The drawing under review shows one solid part. Ordinate dimensions are in mm from its lowest x, y, z. A direction names the side the tool comes from. Coordinates: 2 decimals unless noted, no trailing zeros. Order: outer loops, then holes, each group sorted by start corner. A loop starts at its lowest first (then second) coordinate and runs counter-clockwise, first axis right, second up. Notation, with made-up numbers: (34.25, -36.75) - (85.25, -36.75) arc R16 cw to (85.25, -23.75) - close; hole circle Ø9 at (82, 41.25). An arc over 180 degrees is marked (long way). Answer in a Markdown table with one row per item.
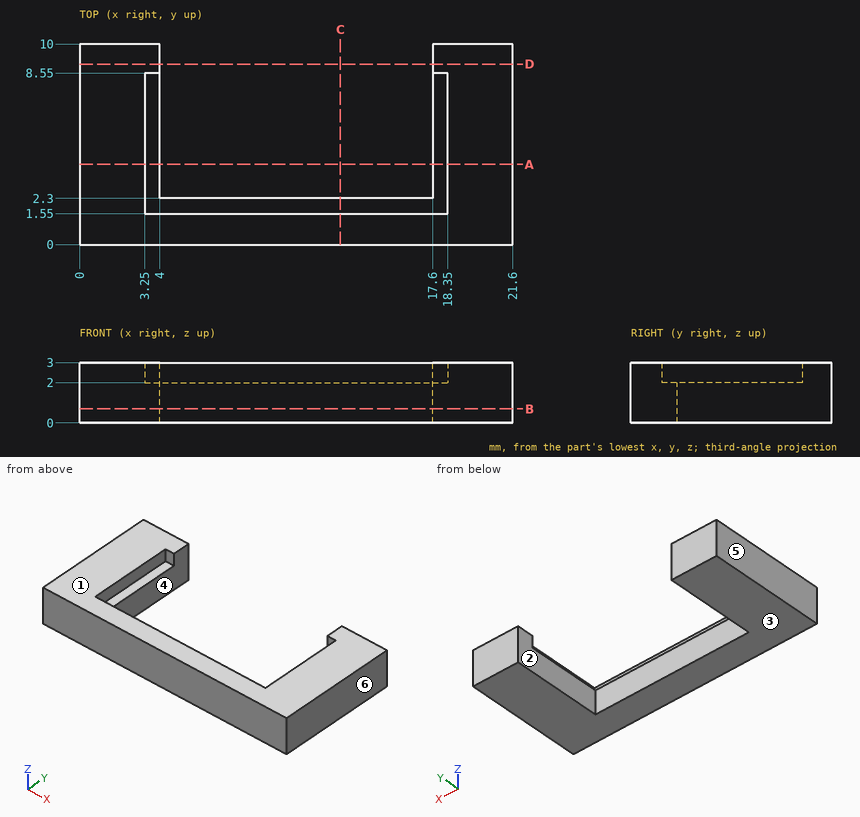
Item 1: Clearance check with a flat-ended pin moving along its axis: pin 1 Ø3.5 at (x, y) = (8.5, 4) entering from +Z. State where the tip first meets the part, or that it passes through.
Check values:
| item | result |
|---|---|
| pin 1 | z = 2 |
Item 2: We need section A-A, the plane y = 4. Write out the cut boundary in (x, z).
Check values:
| item | result |
|---|---|
| outline | (0, 0) - (4, 0) - (4, 2) - (3.25, 2) - (3.25, 3) - (0, 3) - close; (17.6, 0) - (21.6, 0) - (21.6, 3) - (18.35, 3) - (18.35, 2) - (17.6, 2) - close |
Item 3: We need section D-D, the plane y = 9. Write out the cut boundary in (x, z), then the cut area to 3 significant figures.
Check values:
| item | result |
|---|---|
| outline | (0, 0) - (4, 0) - (4, 3) - (0, 3) - close; (17.6, 0) - (21.6, 0) - (21.6, 3) - (17.6, 3) - close |
| area | 24.0 mm^2 |
Item 4: Mouldability with a two-part tool opening along X and no side actions: class the marked faces 3, 4, 5 and 6 as +X half, -X half, draft (parallel to the pull), parting line (faces both ways), or undercut.
Check values:
| item | result |
|---|---|
| face 3 | draft |
| face 4 | undercut |
| face 5 | -X half |
| face 6 | +X half |
Item 5: We need section C-C, the plane x = 13. Write out the cut boundary in (y, z), then the cut area to 3 significant figures.
Check values:
| item | result |
|---|---|
| outline | (0, 0) - (2.3, 0) - (2.3, 2) - (1.55, 2) - (1.55, 3) - (0, 3) - close |
| area | 6.15 mm^2 |
Item 6: To check wall thickness, follow line 1 (X direction, y = 8.75, z = 0.6); line 2 (X direction, y = 3.5, z = 2.4); line 3 (Y direction, x = 10.5, z = 0.3). State the ranges of each line that lie inside material, in increasing order. Write a range as from..to.
Check values:
| item | result |
|---|---|
| line 1 | 0..4, 17.6..21.6 |
| line 2 | 0..3.25, 18.35..21.6 |
| line 3 | 0..2.3 |
Item 7: We need section B-B, the plane z = 0.7. Write out the cut boundary in (x, y), then the cut area to 3 significant figures.
Check values:
| item | result |
|---|---|
| outline | (0, 0) - (21.6, 0) - (21.6, 10) - (17.6, 10) - (17.6, 2.3) - (4, 2.3) - (4, 10) - (0, 10) - close |
| area | 111 mm^2 |
Item 8: Tool access review of the marked faces 1 and 2: name each direction out of +Z, -Z, +X, -X, +Y, -Y from which nothing blocks a thin tool from reaching the whole face with its end or side.
Check values:
| item | result |
|---|---|
| face 1 | +Z, +X, -X, +Y, -Y |
| face 2 | +Z, -Z, +Y |
